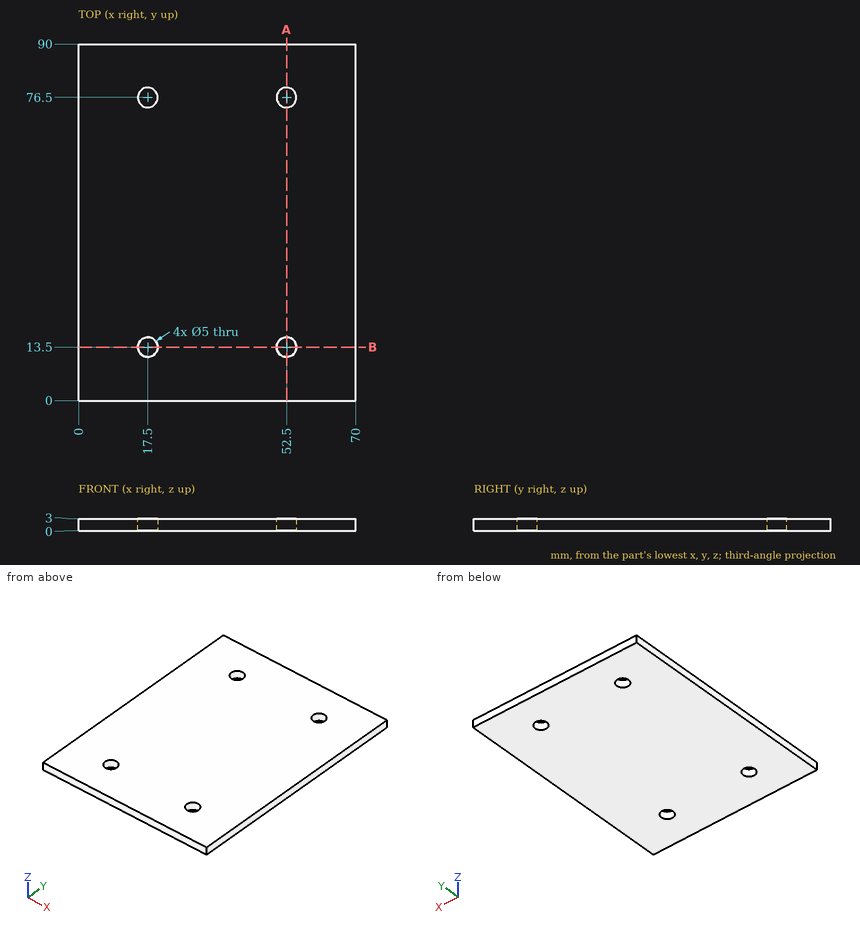
Drawing for the job (mm, zero at the part's lowest x, y, z). Round coordinates to 2 decimals unless told otherwise and drop trailing zeros. Write each loop counter-clockwise with the first axis right and the second up, starting at its lowest first coordinate (ties: lowest second). Pieces come first, ordered by that corner, then holes. Notation, with made-up numbers: (18.5, -17) - (66.5, -17) arc R26 cw to (66.5, 5) - close; hole circle Ø5 at (34.25, 77.5). An arc over 180 degrees is marked (long way). Return JSON: item names as keys, results as strings. Group by question number.
Item 1: Band-saw the part on B-B on y = 13.5. List the corners of the cut face in (x, z).
Item 2: Band-saw the part on A-A on x = 52.5. List the corners of the cut face in (y, z), plus the area to 3 significant figures.
Item 3: Flat gauge pin, fed straight in: pin 1 Ø4.5 at (x, y) = (17.5, 76.5) entering from -Z. Where does the tip first touch, or does it go through?
Item 4: Probe probe 1 along Y at (x, z) = (52.5, 1.95); probe 2 along X at (y, z) = (13.5, 1.5); probe 3 along Y at (x, z) = (53.5, 2.4). List the from-to ranges inside material, lowest first.
Resolved:
{
 "1": {"outline": "(0, 0) - (15, 0) - (15, 3) - (0, 3) - close; (20, 0) - (50, 0) - (50, 3) - (20, 3) - close; (55, 0) - (70, 0) - (70, 3) - (55, 3) - close"},
 "2": {"outline": "(0, 0) - (11, 0) - (11, 3) - (0, 3) - close; (16, 0) - (74, 0) - (74, 3) - (16, 3) - close; (79, 0) - (90, 0) - (90, 3) - (79, 3) - close", "area": "240 mm²"},
 "3": {"pin 1": "passes through"},
 "4": {"probe 1": "y = 0 to 11, 16 to 74, 79 to 90", "probe 2": "x = 0 to 15, 20 to 50, 55 to 70", "probe 3": "y = 0 to 11.21, 15.79 to 74.21, 78.79 to 90"}
}
